```python
from build123d import *

# Parameters (mm, degrees)
SKETCH1_W           = 12.7
SKETCH1_H           = 15.875
BOSS_EXTRUDE1_DEPTH = 1.5875


with BuildPart() as part:
    # Sketch1 → Boss-Extrude1 (new body, symmetric)
    with BuildSketch(Plane.XY):
        with Locations((0, -1.5875)):
            Rectangle(SKETCH1_W, SKETCH1_H)
        Polygon((2.522327856, 4.3688), (-2.522327856, 4.3688), (-5.044655712, 0), (-2.522327856, -4.3688), (2.522327856, -4.3688), (5.044655712, 0), align=None, mode=Mode.SUBTRACT)
    extrude(amount=BOSS_EXTRUDE1_DEPTH, both=True)


solid = part.part
```
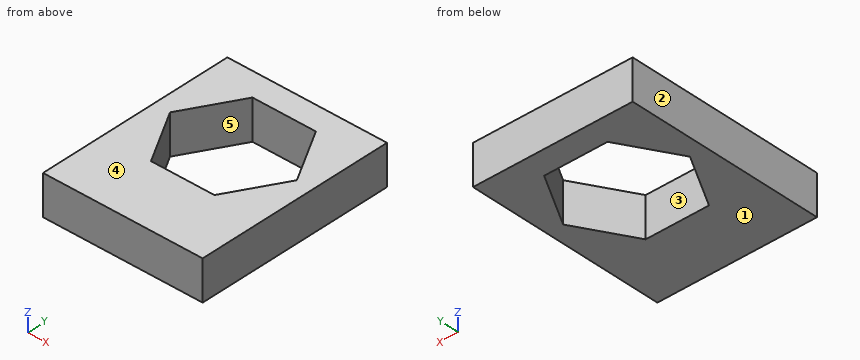
Could you check a few things on this model? Use its own coordinates, in mm. Face numbers are marked on the shaded views. A direction names the side the tool comes from. Round coordinates to 2 decimals unless told otherwise and drop trailing zeros. Write each loop counter-clockwise with the first axis right and the second up, starting at its lowest first coordinate (ties: lowest second). Pieces come first, ordered by that corner, then holes. Notation, with made-up numbers: M -24,9.25 L 8,9.25 A24 cw 8,43.25 Z; hole C -21,18 d11. An arc over 180 degrees is marked long. Write each question's results on one line, items separated by ' | '. Start each with the question number.
1. I need wall thicknesses on L1, parallel to Y at x = 0.5, z = -0.9 (3 decimals); L2, parallel to X at y = -2.25, z = 0.1; L3, parallel to Y at x = 4.25, z = 0.1 (3 decimals). Which ranges of each line are inside material? Lowest first, please. Write a range as from..to.
2. On a 3-axis mill with a long thin cutter (end or side, diameter ignored), from which of +Z, -Z, +X, -X, +Y, -Y can I reach the whole of each face in a straight line? I mean the marked faces 4 and 5. Say none if no direction works.
3. Thinking about a two-plate mould opening in X: for the marked faces 1, 2 and 3, which applies, +X half, -X half, draft (parallel to the pull), parting line (faces both ways), or undercut?
4. Imagine slicing it at B-B on y = -4. List the corners of the cut face in (x, z) for me.
5. Imagine slicing it at A-A on z = 0.8. List the corners of the cut face in (x, y) for me (3 decimals).
Result sheet:
1) L1: y = -9.525..-4.369, 4.369..6.35 | L2: x = -6.35..-3.75, 3.75..6.35 | L3: y = -9.525..-1.376, 1.376..6.35
2) face 4: +Z, +X, -X, +Y, -Y | face 5: +Z, -Z
3) face 1: draft | face 2: -X half | face 3: undercut
4) outline: M -6.35,-1.59 L -2.74,-1.59 L -2.74,1.59 L -6.35,1.59 Z; M 2.74,-1.59 L 6.35,-1.59 L 6.35,1.59 L 2.74,1.59 Z
5) outline: M -6.35,-9.525 L 6.35,-9.525 L 6.35,6.35 L -6.35,6.35 Z; hole M -5.045,0 L -2.522,-4.369 L 2.522,-4.369 L 5.045,0 L 2.522,4.369 L -2.522,4.369 Z
